Design review of the part built by this model. Coordinates are the model's own, in mm. A direction names the side the tool comes from. Give positions to 0.01 mm unless a question says otherwise; leave off trailing zeros. Write each loop counter-clockwise with the first axis right and the second up, starting at its lowest first coordinate (ties: lowest second). Pieces come first, ordered by that corner, then holes. Notation, with made-up numbers: M -33,-8.5 L 8,-8.5 A24 cw 8,24.5 Z; hole C 68,78.5 d10. An arc over 180 degrees is marked long. Answer in a Markdown table with one row per item.
```python
from build123d import *

# Parameters (mm, degrees)
F1_DEPTH = 12.7
F2_DEPTH = 95.25


# Not quite as in the source:
# - a feature names something its author has since deleted; it is built from what else it names


with BuildPart() as f1:
    # F0 (on Front) → F1 (new body)
    with BuildSketch(Plane.XZ):
        Polygon((-22.6091385288, 130.2924993012), (-4.278267482, 98.5424993012), (32.3834746115, 98.5424993012), (50.7143456583, 130.2924993012), (32.3834746116, 162.0424993012), (-4.278267482, 162.0424993012), align=None)
        Polygon((-2.4451803773, 101.7174993012), (-18.9429643194, 130.2924993012), (-2.4451803773, 158.8674993012), (30.5503875069, 158.8674993012), (47.048171449, 130.2924993012), (30.5503875069, 101.7174993012), align=None, mode=Mode.SUBTRACT)
        Polygon((-27.4963065598, 130.2924993012), (-22.6091385288, 130.2924993012), (-4.278267482, 162.0424993012), (-22.6091385288, 193.7924993012), (-59.2708806223, 193.7924993012), (-77.6017516691, 162.0424993012), (-59.2708806223, 130.2924993012), align=None)
        Polygon((-57.4377935176, 133.4674993012), (-73.9355774597, 162.0424993012), (-57.4377935176, 190.6174993012), (-24.4422256334, 190.6174993012), (-7.9444416913, 162.0424993012), (-24.4422256334, 133.4674993012), align=None, mode=Mode.SUBTRACT)
        Polygon((32.3834746116, 162.0424993012), (50.7143456583, 130.2924993012), (87.3760877519, 130.2924993012), (105.7069587986, 162.0424993012), (87.3760877519, 193.7924993012), (50.7143456583, 193.7924993012), align=None)
        Polygon((52.547432763, 133.4674993012), (36.0496488209, 162.0424993012), (52.547432763, 190.6174993012), (85.5430006472, 190.6174993012), (102.0407845893, 162.0424993012), (85.5430006472, 133.4674993012), align=None, mode=Mode.SUBTRACT)
        Polygon((-57.4377935176, 190.6174993012), (-73.9355774597, 162.0424993012), (-57.4377935176, 133.4674993012), (-24.4422256334, 133.4674993012), (-7.9444416913, 162.0424993012), (-24.4422256334, 190.6174993012), align=None)
        Polygon((52.547432763, 190.6174993012), (36.0496488209, 162.0424993012), (52.547432763, 133.4674993012), (85.5430006472, 133.4674993012), (102.0407845893, 162.0424993012), (85.5430006472, 190.6174993012), align=None)
        Polygon((-2.4451803773, 158.8674993012), (-18.9429643194, 130.2924993012), (-2.4451803773, 101.7174993012), (30.5503875069, 101.7174993012), (47.048171449, 130.2924993012), (30.5503875069, 158.8674993012), align=None)
    extrude(amount=F1_DEPTH)

    # F0 (on Front) → F2 (join)
    with BuildSketch(Plane.XZ):
        Polygon((-22.6091385288, 130.2924993012), (-4.278267482, 98.5424993012), (32.3834746115, 98.5424993012), (50.7143456583, 130.2924993012), (32.3834746116, 162.0424993012), (-4.278267482, 162.0424993012), align=None)
        Polygon((-2.4451803773, 101.7174993012), (-18.9429643194, 130.2924993012), (-2.4451803773, 158.8674993012), (30.5503875069, 158.8674993012), (47.048171449, 130.2924993012), (30.5503875069, 101.7174993012), align=None, mode=Mode.SUBTRACT)
        Polygon((32.3834746116, 162.0424993012), (50.7143456583, 130.2924993012), (87.3760877519, 130.2924993012), (105.7069587986, 162.0424993012), (87.3760877519, 193.7924993012), (50.7143456583, 193.7924993012), align=None)
        Polygon((52.547432763, 133.4674993012), (36.0496488209, 162.0424993012), (52.547432763, 190.6174993012), (85.5430006472, 190.6174993012), (102.0407845893, 162.0424993012), (85.5430006472, 133.4674993012), align=None, mode=Mode.SUBTRACT)
        Polygon((-27.4963065598, 130.2924993012), (-22.6091385288, 130.2924993012), (-4.278267482, 162.0424993012), (-22.6091385288, 193.7924993012), (-59.2708806223, 193.7924993012), (-77.6017516691, 162.0424993012), (-59.2708806223, 130.2924993012), align=None)
        Polygon((-57.4377935176, 133.4674993012), (-73.9355774597, 162.0424993012), (-57.4377935176, 190.6174993012), (-24.4422256334, 190.6174993012), (-7.9444416913, 162.0424993012), (-24.4422256334, 133.4674993012), align=None, mode=Mode.SUBTRACT)
        Polygon((-22.6091385288, 193.7924993012), (-4.278267482, 162.0424993012), (32.3834746116, 162.0424993012), (50.7143456583, 193.7924993012), (87.3760877519, 193.7924993012), (105.7069587986, 162.0424993012), (87.3760877519, 130.2924993012), (91.0422619612, 130.2924993012), (109.373133008, 162.0424993012), (89.2091748565, 196.9674993012), (48.8812585537, 196.9674993012), (30.5503875069, 165.2174993012), (-2.4451803773, 165.2174993012), (-20.7760514241, 196.9674993012), (-61.103967727, 196.9674993012), (-79.4348387737, 165.2174993012), (-77.6017516691, 162.0424993012), (-59.2708806223, 193.7924993012), align=None)
        Polygon((-7.9444416913, 98.5424993012), (-4.278267482, 98.5424993012), (-22.6091385288, 130.2924993012), (-27.4963065598, 130.2924993012), (-59.2708806223, 130.2924993012), (-57.4377935176, 127.1174993012), (-24.4422256334, 127.1174993012), align=None)
    extrude(amount=F2_DEPTH)


solid = f1.part
```
1) For faces 1 (the face through (99.432, -46.958, 179.261)), 2 (the face through (93.91, -53.4, 147.96)), 3 (the face through (-41, -47, 127.117)), 4 (the face through (39.84, -46.96, 181.31)), 5 (the face through (100.08, -46.96, 145.95)), list the 3-axis set-ups (+Z, -Z, +X, -X, +Y, -Y) from which the entire face can be reached by the end or side of a thin tool; tool diameter is ignored.
Geometry says:
| item | result |
|---|---|
| face 1 | +Z, +X, +Y, -Y |
| face 2 | -Y |
| face 3 | -Z, -X, +Y, -Y |
| face 4 | +Z, +Y, -Y |
| face 5 | -Z, +X, +Y, -Y |
2) Add section A-A (x = -52.5). Write out the cut boundary in (y, z).
Geometry says:
| item | result |
|---|---|
| outline | M -95.25,127.12 L 0,127.12 L 0,196.97 L -95.25,196.97 L -95.25,190.62 L -12.7,190.62 L -12.7,133.47 L -95.25,133.47 Z |
3) The part is to be moulded in two halves that separate along Z. For faces 6 (the face through (14, -53, 158.867)), 7 (the face through (71, -47, 130.292)), 8 (the face through (14, 0, 148)), say which applies: released by +Z, released by -Z, zero draft, split by the parting line, or undercut.
Geometry says:
| item | result |
|---|---|
| face 6 | undercut |
| face 7 | released by -Z |
| face 8 | zero draft |
4) Add section C-C (z = 116). Write out the cut boundary in (x, y), and give its area (3 significant figures).
Geometry says:
| item | result |
|---|---|
| outline | M -18.02,-95.25 L -10.69,-95.25 L -10.69,-12.7 L 38.8,-12.7 L 38.8,-95.25 L 42.46,-95.25 L 42.46,0 L -18.02,0 Z |
| area | 1,680 mm^2 |
5) Add section D-D (x = -15). Write out the cut boundary in (y, z).
Geometry says:
| item | result |
|---|---|
| outline | M -95.25,110.76 L 0,110.76 L 0,186.96 L -95.25,186.96 L -95.25,174.26 L -12.7,174.26 L -12.7,149.82 L -95.25,149.82 L -95.25,137.12 L -12.7,137.12 L -12.7,123.46 L -95.25,123.46 Z |
6) To check wall thickness, follow probe 1 along Z at (x, y) = (-32, -58); probe 2 along X at (y, z) = (-56, 144); probe 3 along Z at (x, y) = (1.5, -80.5). State the ranges of each line that lie inside material, in increasing order. Write a range as [from, to].
Geometry says:
| item | result |
|---|---|
| probe 1 | [127.12, 133.47], [190.62, 196.97] |
| probe 2 | [-67.18, -63.52], [-18.36, -11.03], [39.13, 46.47], [91.62, 98.96] |
| probe 3 | [98.54, 101.72], [158.87, 165.22] |
7) Insertion check: P1, Ø16.5, axis at x = -36, y = -61, coming from the -Z side; P2, Ø3, axis at x = 26.5, z = 132.5, coming from the +Y side; P3, Ø3, axis at y = -27, z = 133, coming from the -X side; P4, Ø10, axis at y = -9.5, z = 172, coming from the -X side. Each pin has a flat end and moves straight along its axis. Give the tip position at first contact, or say it passes through.
Geometry says:
| item | result |
|---|---|
| P1 | z = 127.12 |
| P2 | y = 0 |
| P3 | x = -61.7 |
| P4 | x = -78.41 |
8) Add section B-B (y = -22). Count the separate pieces of the cut face and the enclosed holes in it, and give its area (3 significant figures).
Geometry says:
| item | result |
|---|---|
| separate pieces | 1 |
| enclosed holes | 3 |
| area | 3,150 mm^2 |
